from build123d import *

# Parameters (mm, degrees)
SKETCH1_W                      = 254
SKETCH1_H                      = 114.3
BOSS_EXTRUDE1_DEPTH            = 9.525
F_3_8_CLEARANCE_HOLE1_D        = 9.8044
F_3_8_CLEARANCE_HOLE1_DEPTH    = 10
F_3_8_CLEARANCE_HOLE1_TIP      = 2.945538927
M2_5_CLEARANCE_HOLE3_D         = 3.3
M2_5_CLEARANCE_HOLE3_DEPTH     = 10
M2_5_CLEARANCE_HOLE3_TIP       = 0.991420021
FILLET1_R                      = 2
M3_CLEARANCE_HOLE4_D           = 4.45
M3_CLEARANCE_HOLE4_DEPTH       = 10
M3_CLEARANCE_HOLE4_TIP         = 1.336914877
SKETCH22_R                     = 8
CUT_EXTRUDE1_DEPTH             = 140.5917194
M3_CLEARANCE_HOLE5_D           = 4.45
M3_CLEARANCE_HOLE5_DEPTH       = 10
M3_CLEARANCE_HOLE5_TIP         = 1.336914877
M2_5_CLEARANCE_HOLE4_OUTLINE_R = 1.65
M2_5_CLEARANCE_HOLE4_DEPTH     = 9.525


# Read off the part's stored shape, not the designer's step: M2.5 Clearance Hole4
with BuildPart() as part:
    # Sketch1 → Boss-Extrude1 (new body)
    with BuildSketch(Plane(origin=(0, 0, 0), x_dir=(1, 0, 0), z_dir=(0, 1, 0))):
        Rectangle(SKETCH1_W, SKETCH1_H)
    extrude(amount=BOSS_EXTRUDE1_DEPTH)

    # 3/8 Clearance Hole1
    with Locations(Plane(origin=(0, 9.525, 0), x_dir=(1, 0, 0), z_dir=(0, 1, 0))):
        with Locations((112.7125, 42.8625), (112.7125, -42.8675), (-112.7175, 42.8625), (-112.7175, -42.8675)):
            Hole(F_3_8_CLEARANCE_HOLE1_D / 2, depth=F_3_8_CLEARANCE_HOLE1_DEPTH)
            with Locations((0, 0, -(F_3_8_CLEARANCE_HOLE1_DEPTH + F_3_8_CLEARANCE_HOLE1_TIP / 2))):  # 118° drill point
                Cone(0, F_3_8_CLEARANCE_HOLE1_D / 2, F_3_8_CLEARANCE_HOLE1_TIP, mode=Mode.SUBTRACT)

    # M2.5 Clearance Hole3
    with Locations(Plane(origin=(0, 9.525, 0), x_dir=(1, 0, 0), z_dir=(0, 1, 0))):
        with Locations((24.5, 19), (-24.5, -39), (24.5, -39), (-24.5, 19)):
            Hole(M2_5_CLEARANCE_HOLE3_D / 2, depth=M2_5_CLEARANCE_HOLE3_DEPTH)
            with Locations((0, 0, -(M2_5_CLEARANCE_HOLE3_DEPTH + M2_5_CLEARANCE_HOLE3_TIP / 2))):  # 118° drill point
                Cone(0, M2_5_CLEARANCE_HOLE3_D / 2, M2_5_CLEARANCE_HOLE3_TIP, mode=Mode.SUBTRACT)

    # Fillet1
    fillet1_edges = [part.edges().sort_by_distance(p)[0] for p in [
        (127, 4.7625, 57.15),
        (-127, 4.7625, 57.15),
        (-127, 4.7625, -57.15),
        (127, 4.7625, -57.15),
    ]]
    fillet(fillet1_edges, radius=FILLET1_R)

    # M3 Clearance Hole4
    with Locations(Plane(origin=(0, 9.525, 0), x_dir=(1, 0, 0), z_dir=(0, 1, 0))):
        with Locations((-58.8, 29.15), (-46, -20.8), (-90.2, -20.8), (-88.35, 13.25)):
            Hole(M3_CLEARANCE_HOLE4_D / 2, depth=M3_CLEARANCE_HOLE4_DEPTH)
            with Locations((0, 0, -(M3_CLEARANCE_HOLE4_DEPTH + M3_CLEARANCE_HOLE4_TIP / 2))):  # 118° drill point
                Cone(0, M3_CLEARANCE_HOLE4_D / 2, M3_CLEARANCE_HOLE4_TIP, mode=Mode.SUBTRACT)

    # Sketch22 → Cut-Extrude1 (cut, through all)
    with BuildSketch(Plane(origin=(0, 9.525, 0), x_dir=(1, 0, 0), z_dir=(0, 1, 0))):
        with Locations(Location((-107.475, 0, 0), (0, 0, 270))):
            Circle(SKETCH22_R)
    extrude(amount=-CUT_EXTRUDE1_DEPTH, mode=Mode.SUBTRACT)

    # M3 Clearance Hole5
    with Locations(Plane(origin=(0, 9.525, 0), x_dir=(1, 0, 0), z_dir=(0, 1, 0))):
        with Locations((61.84, 40.64), (61.84, -40.64), (82.16, -40.64), (82.16, 40.64)):
            Hole(M3_CLEARANCE_HOLE5_D / 2, depth=M3_CLEARANCE_HOLE5_DEPTH)
            with Locations((0, 0, -(M3_CLEARANCE_HOLE5_DEPTH + M3_CLEARANCE_HOLE5_TIP / 2))):  # 118° drill point
                Cone(0, M3_CLEARANCE_HOLE5_D / 2, M3_CLEARANCE_HOLE5_TIP, mode=Mode.SUBTRACT)

    # M2.5 Clearance Hole4 outline → M2.5 Clearance Hole4 (cut)
    with BuildSketch(Plane(origin=(0, 0, 0), x_dir=(1, 0, 0), z_dir=(0, 1, 0))):
        with Locations((-10.16, 6.35)):
            Circle(M2_5_CLEARANCE_HOLE4_OUTLINE_R)
        with Locations((10.16, 6.35)):
            Circle(M2_5_CLEARANCE_HOLE4_OUTLINE_R)
        with Locations((10.16, -6.35)):
            Circle(M2_5_CLEARANCE_HOLE4_OUTLINE_R)
        with Locations((-10.16, -6.35)):
            Circle(M2_5_CLEARANCE_HOLE4_OUTLINE_R)
    extrude(amount=M2_5_CLEARANCE_HOLE4_DEPTH, mode=Mode.SUBTRACT)


solid = part.part
The listing builds one solid part. Answer for the finished solid, in the listing's coordinates (mm). Give positions to 0.01 mm unless a question says otherwise; leave off trailing zeros. Answer as a JSON object with one key per item and string values.
1. Find the intervals of material crossed by L1, parallel to Z at x = 24.5, y = 5.75; L2, parallel to X at y = 4.25, z = -19; L3, parallel to Z at x = 10.16, y = 2, in increasing order. Write a range as [from, to].
Determined:
{"L1": "[-57.15, -20.65], [-17.35, 37.35], [40.65, 57.15]", "L2": "[-127, -26.15], [-22.85, 22.85], [26.15, 127]", "L3": "[-57.15, -8], [-4.7, 4.7], [8, 57.15]"}
2. A flat-ended cylindrical pin translates along its axis: pin 1 Ø5 at (x, z) = (-58, -32.5) entering from -Y. Find the tip coordinate at first contact, or state that the pin passes through.
Determined:
{"pin 1": "y = 0"}
3. A cutting plane is placed at A-A (y = 3). Give the number of separate pieces and of enclosed holes in the cut face, then the cut area to 3 significant figures.
Determined:
{"separate pieces": "1", "enclosed holes": "21", "area": "28,300 mm²"}
4. For a pull along Z with two mould halves and no side action, classify faces 1 (the cylindrical face through (-47.196, 4.696, 18.924)), 2 (the flat face through (-127, 5, 1)), 3 (the flat face through (-2, 5, -57.15)) as pulls with the +Z half, pulls with the -Z half, needs draft (parallel to the pull), parting line crosses it, or undercut.
Determined:
{"face 1": "undercut", "face 2": "needs draft", "face 3": "pulls with the -Z half"}
